Check sheet for the modelled part. Datum: model origin and axes. Units: mm. A direction names the side the tool comes from. Round coordinates to 2 decimals unless told otherwise and drop trailing zeros. Loops run counter-clockwise (first coordinate to the right, second up) from the corner with the lowest first, then second, coordinate; pieces in that order, holes last. Notation, with made-up numbers: (12, -31) - (59, -31) arc R16 ccw to (59, -24) - close; hole circle Ø3 at (58.5, 13). An arc over 180 degrees is marked (long way). Put each result on its own line as item: value.
```python
from build123d import *

# Parameters (mm, degrees)
BOSS_EXTRUDE1_DEPTH = 50
CUT_EXTRUDE2_DEPTH  = 4
CUT_EXTRUDE5_DEPTH  = 2
CUT_EXTRUDE7_DEPTH  = 20
CUT_EXTRUDE9_DEPTH  = 25
CUT_EXTRUDE14_DEPTH = 6
HOLE1_D             = 6
SKETCH18_W          = 25
SKETCH18_H          = 6
CUT_EXTRUDE15_DEPTH = 5


with BuildPart() as part:
    # Sketch1 → Boss-Extrude1 (new body)
    with BuildSketch(Plane(origin=(0, 0, 0), x_dir=(1, 0, 0), z_dir=(0, 1, 0))):
        with BuildLine():
            Line((-360, 39.99999406), (360, 39.99999406))
            ThreePointArc((360, 39.99999406), (399.999998105, -4.045e-06), (360, -40))
            Line((360, -40), (-360, -40))
            ThreePointArc((-360, -40), (-399.99999406, -5.94e-06), (-360, 39.99999406))
        make_face()
    extrude(amount=BOSS_EXTRUDE1_DEPTH)

    # Sketch4 → Cut-Extrude2 (cut)
    with BuildSketch(Plane.XZ):
        with BuildLine():
            Line((360, 35.000001075), (-360, 35.000001485))
            ThreePointArc((-360, 35.000001485), (-394.999995545, 5.94e-06), (-360, -34.999989605))
            Line((-360, -34.999989605), (360.000000021, -34.99999406))
            ThreePointArc((360.000000021, -34.99999406), (394.999998105, 4.055e-06), (360, 35.000001075))
        make_face()
    extrude(amount=-CUT_EXTRUDE2_DEPTH, mode=Mode.SUBTRACT)

    # Sketch6 → Cut-Extrude5 (cut)
    with BuildSketch(Plane(origin=(0, 50, 0), x_dir=(1, 0, 0), z_dir=(0, 1, 0))):
        with BuildLine():
            Line((360.000000021, 34.99999406), (117.999999967, 34.999993062))
            ThreePointArc((117.999999967, 34.999993062), (112.343145739, 32.6568473), (110, 26.999993062))
            Line((110, 26.999993062), (110, -27))
            ThreePointArc((110, -27), (112.343145751, -32.656854249), (118, -35))
            Line((118, -35), (360, -35))
            ThreePointArc((360, -35), (394.999995955, -4.055e-06), (360.000000021, 34.99999406))
        make_face()
    extrude(amount=-CUT_EXTRUDE5_DEPTH, mode=Mode.SUBTRACT)

    # Sketch7 → Cut-Extrude7 (cut)
    with BuildSketch(Plane(origin=(0, 48, 0), x_dir=(1, 0, 0), z_dir=(0, 1, 0))):
        with BuildLine():
            Line((122, 26.999992985), (356, 26.999992985))
            ThreePointArc((356, 26.999992985), (358.828427125, 25.82842011), (360, 22.999992985))
            Line((360, 22.999992985), (360, -23))
            ThreePointArc((360, -23), (358.828427125, -25.828427125), (356, -27))
            Line((356, -27), (122, -27))
            ThreePointArc((122, -27), (119.171572875, -25.828427125), (118, -23))
            Line((118, -23), (118, 22.999992985))
            ThreePointArc((118, 22.999992985), (119.171572875, 25.82842011), (122, 26.999992985))
        make_face()
    extrude(amount=-CUT_EXTRUDE7_DEPTH, mode=Mode.SUBTRACT)

    # Sketch2 → Cut-Extrude9 (cut)
    with BuildSketch(Plane.XZ.offset(-4)):
        with BuildLine():
            Line((356, 27), (-356, 27))
            ThreePointArc((-356, 27), (-358.828427125, 25.828427125), (-360, 23))
            Line((-360, 23), (-360, -22.99999406))
            ThreePointArc((-360, -22.99999406), (-358.828427125, -25.828421185), (-356, -26.99999406))
            Line((-356, -26.99999406), (356, -26.99999406))
            ThreePointArc((356, -26.99999406), (358.828427125, -25.828421185), (360, -22.99999406))
            Line((360, -22.99999406), (360, 23))
            ThreePointArc((360, 23), (358.828427125, 25.828427125), (356, 27))
        make_face()
    extrude(amount=-CUT_EXTRUDE9_DEPTH, mode=Mode.SUBTRACT)

    # Sketch15 → Cut-Extrude14 (cut)
    with BuildSketch(Plane.XZ.offset(-4)):
        with BuildLine():
            Line((-360, -30), (360, -30))
            ThreePointArc((360, -30), (364, -26), (360, -22))
            Line((360, -22), (360, -22.99999406))
            ThreePointArc((360, -22.99999406), (358.828427125, -25.828421185), (356, -26.99999406))
            Line((356, -26.99999406), (-356, -26.99999406))
            ThreePointArc((-356, -26.99999406), (-358.828427125, -25.828421185), (-360, -22.99999406))
            Line((-360, -22.99999406), (-360, -22))
            ThreePointArc((-360, -22), (-364, -26), (-360, -30))
        make_face()
        with BuildLine():
            Line((360, 23), (360, 22))
            ThreePointArc((360, 22), (364, 26), (360, 30))
            Line((360, 30), (-360, 30))
            ThreePointArc((-360, 30), (-364, 26), (-360, 22))
            Line((-360, 22), (-360, 23))
            ThreePointArc((-360, 23), (-358.828427125, 25.828427125), (-356, 27))
            Line((-356, 27), (356, 27))
            ThreePointArc((356, 27), (358.828427125, 25.828427125), (360, 23))
        make_face()
    extrude(amount=-CUT_EXTRUDE14_DEPTH, mode=Mode.SUBTRACT)

    # Hole1 (through all)
    with Locations(Plane(origin=(0, 4, 0), x_dir=(-1, 0, 0), z_dir=(0, -1, 0))):
        with Locations((-385, 0)):
            Hole(HOLE1_D / 2)

    # Sketch18 → Cut-Extrude15 (cut)
    with BuildSketch(Plane(origin=(0, 48, 0), x_dir=(1, 0, 0), z_dir=(0, 1, 0))):
        with Locations((372.5, 0)):
            Rectangle(SKETCH18_W, SKETCH18_H)
    extrude(amount=-CUT_EXTRUDE15_DEPTH, mode=Mode.SUBTRACT)


solid = part.part
```
Item 1: Release check for a two-part mould opening along X. For faces 5 (the cylindrical face through (-399.99, 24.65, 0.88)), 6 (the flat face through (5, 25, 40)), 7 (the flat face through (-5, 19, -27)), 8 (the flat face through (118, 39, 0)) record: +X half, -X half, draft (parallel to the pull), parting line (faces both ways), or undercut.
Filled sheet:
face 5: -X half
face 6: draft
face 7: undercut
face 8: undercut
Item 2: Go/stop test with flat-tipped pins: pin 1 (12 mm diameter, centred on x = -169.5, z = -26.5, fed in from -Y); pin 2 (9.5 mm diameter, centred on y = 42.5, z = 2, fed in from +X); pin 3 (3 mm diameter, centred on x = -273.5, z = -16.5, fed in from -Y). Record where each tip stops, or that it passes through.
Filled sheet:
pin 1: y = 4
pin 2: x = 400
pin 3: y = 29
Item 3: Thickness scan on line 1 (Z direction, x = 40, y = 9); line 2 (Z direction, x = 227, y = 19); line 3 (X direction, y = 22, z = -1). Record the ranges inside material, lowest first. Write a range as from..to.
Filled sheet:
line 1: -40..-30, 30..40
line 2: -40..-27, 27..40
line 3: -399.99..-360, 360..382.17, 387.83..399.99
Item 4: Section check B-B on x = 96. Enter the section's corners in (y, z), then the cut area to 3 significant figures.
Filled sheet:
outline: (0, -40) - (50, -40) - (50, 40) - (0, 40) - (0, 35) - (4, 35) - (4, 30) - (10, 30) - (10, 27) - (29, 27) - (29, -27) - (10, -27) - (10, -30) - (4, -30) - (4, -35) - (0, -35) - close
area: 2,330 mm²
Item 5: Section check C-C on y = 20. Enter the section's corners in (x, z).
Filled sheet:
outline: (-360, -40) - (360, -40) arc R40 ccw to (360, 40) - (-360, 40) arc R40 ccw to start; hole (-360, -23) arc R4 ccw to (-356, -27) - (356, -27) arc R4 ccw to (360, -23) - (360, 23) arc R4 ccw to (356, 27) - (-356, 27) arc R4 ccw to (-360, 23) - close; hole circle Ø6 at (385, 0)
Item 6: Tool access check on faces 1 (the flat face through (262, 48, 28)), 2 (the flat face through (237, 39, -27)), 3 (the flat face through (-5, 25, -40)), 4 (the flat face through (-85, 29, 0)). Record the directions out of +Z, -Z, +X, -X, +Y, -Y that give a thin tool (end or side, any length) a straight path to the whole face; none if there is none.
Filled sheet:
face 1: +Y
face 2: +Y, -Y
face 3: -Z, +X, -X, +Y, -Y
face 4: -Y
